Here's the drawing with two shaded views (mm, measured from the low corner). I have some questions. A direction names the side the tool comes from. Coordinates: 2 decimals unless noted, no trailing zeros. Write each loop counter-clockwise with the first axis right and the second up, starting at its lowest first coordinate (ties: lowest second). Pieces come first, ordered by that corner, then holes.
Item 1: I want a section at D-D on y = 7. Please give me the cut outline in (x, z).
Item 2: I want a section at C-C on z = 13.75. Please give me the cut outline in (x, y).
Item 3: For P1, Ø11, axis at y = 38, z = 11, coming from the +X side; P2, Ø10, axis at x = 4.5, y = 34, coming from the +Z side; P3, Ø3, axis at y = 21, z = 3, coming from the +X side; P4, Ø5.5, axis at x = 11, z = 18.5, coming from the -Y side, each with a flat end and sliding along its axis, tell me the tip position at first contact or that it passes through.
Item 4: I want a section at A-A on y = 25. Please give me the cut outline in (x, z).
Item 5: Which directions (+Z, -Z, +X, -X, +Y, -Y) give clear straight access to the entire face, cutting with the end or side of a thin tool? Please do the marked faces 5, 6, 7, 8 and 9.
Item 6: Thinking about a two-plate mould opening in X: for the marked faces 1, 2, 3 and 4, which applies, +X half, -X half, draft (parallel to the pull), parting line (faces both ways), or undercut?
Item 7: If I drill on probe 1 along Y at (x, z) = (17.75, 10.25); probe 2 along X at (y, z) = (7, 13.5); probe 3 along X at (y, z) = (12, 12.25), over which ranges is the centre line in solid material (lowest first)?
Item 8: I want a section at B-B on x = 12.5. Please give me the cut outline in (y, z).
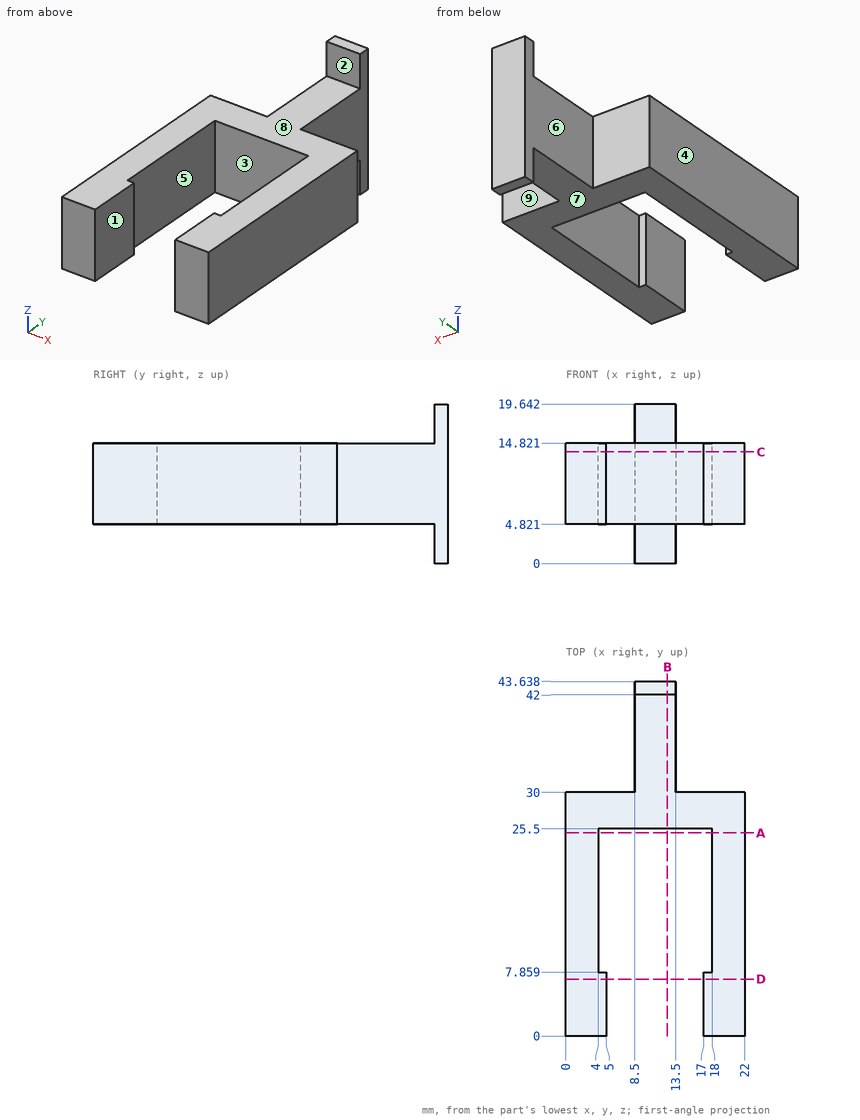
Response values:
1. outline: (0, 4.82) - (5, 4.82) - (5, 14.82) - (0, 14.82) - close; (17, 4.82) - (22, 4.82) - (22, 14.82) - (17, 14.82) - close
2. outline: (0, 0) - (5, 0) - (5, 7.86) - (4, 7.86) - (4, 25.5) - (18, 25.5) - (18, 7.86) - (17, 7.86) - (17, 0) - (22, 0) - (22, 30) - (13.5, 30) - (13.5, 43.64) - (8.5, 43.64) - (8.5, 30) - (0, 30) - close
3. P1: stops at x = 13.5
3. P2: stops at z = 14.82
3. P3: passes through
3. P4: stops at y = 42
4. outline: (0, 4.82) - (4, 4.82) - (4, 14.82) - (0, 14.82) - close; (18, 4.82) - (22, 4.82) - (22, 14.82) - (18, 14.82) - close
5. face 5: +Z, -Z
5. face 6: +Z, -Z, -X, +Y
5. face 7: -Z, +X, -X, -Y
5. face 8: +Z, +X, -X, -Y
5. face 9: +Z, -Z, +X, +Y
6. face 1: undercut
6. face 2: draft
6. face 3: undercut
6. face 4: -X half
7. probe 1: y = 0 to 7.86, 25.5 to 30
7. probe 2: x = 0 to 5, 17 to 22
7. probe 3: x = 0 to 4, 18 to 22
8. outline: (25.5, 4.82) - (42, 4.82) - (42, 0) - (43.64, 0) - (43.64, 19.64) - (42, 19.64) - (42, 14.82) - (25.5, 14.82) - close
